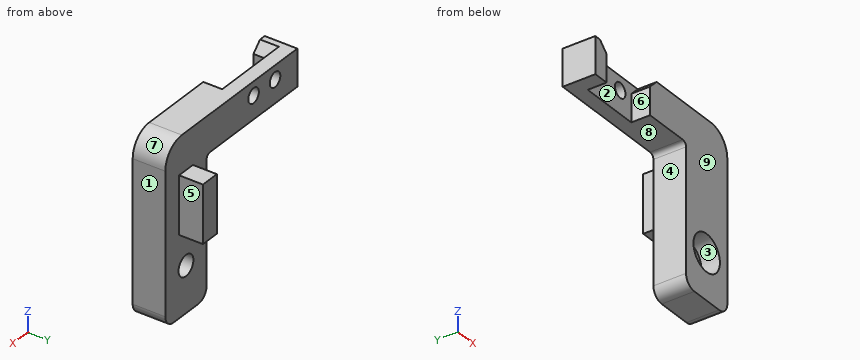
from build123d import *

# Parameters (mm, degrees)
BOSS_EXTRUDE1_DEPTH            = 7.1
SKETCH2_W                      = 4.2
SKETCH2_H                      = 12.5
BOSS_EXTRUDE2_DEPTH            = 5.2
CBORE_FOR_M4_SHCS1_D           = 4.5
CBORE_FOR_M4_SHCS1_CBORE_D     = 8
CBORE_FOR_M4_SHCS1_CBORE_DEPTH = 4
F_3_2_3_2_DIAMETER_HOLE1_D     = 3.2
SKETCH7_W                      = 13.2
SKETCH7_H                      = 8
CUT_EXTRUDE1_DEPTH             = 4.1
FILLET1_R                      = 5
FILLET2_R                      = 2.5
FILLET3_R                      = 1
CHAMFER1_SIZE                  = 2


with BuildPart() as part:
    # Sketch1 → Boss-Extrude1 (new body)
    with BuildSketch(Plane(origin=(0, 0, 0), x_dir=(1, 0, 0), z_dir=(0, 1, 0))):
        Polygon((0, 0), (-12.5, 0), (-12.5, -30), (-40, -30), (-40, -38), (-12.5, -38), (0, -38), align=None)
    extrude(amount=BOSS_EXTRUDE1_DEPTH)

    # Sketch2 → Boss-Extrude2 (add)
    with BuildSketch(Plane(origin=(0, 7.1, 0), x_dir=(1, 0, 0), z_dir=(0, 1, 0))):
        with Locations((-6.25, -23.75)):
            Rectangle(SKETCH2_W, SKETCH2_H)
    extrude(amount=BOSS_EXTRUDE2_DEPTH)

    # CBORE for M4 SHCS1 (through all)
    with Locations(Plane.XZ):
        with Locations((-6.25, 10)):
            CounterBoreHole(CBORE_FOR_M4_SHCS1_D / 2, CBORE_FOR_M4_SHCS1_CBORE_D / 2, CBORE_FOR_M4_SHCS1_CBORE_DEPTH)

    # Ø3.2 (3.2) Diameter Hole1 (through all)
    with Locations(Plane.XZ):
        with Locations((-33.25, 35), (-26.75, 35)):
            Hole(F_3_2_3_2_DIAMETER_HOLE1_D / 2)

    # Sketch7 → Cut-Extrude1 (cut)
    with BuildSketch(Plane.XZ):
        with Locations((-30, 34)):
            Rectangle(SKETCH7_W, SKETCH7_H)
    extrude(amount=-CUT_EXTRUDE1_DEPTH, mode=Mode.SUBTRACT)

    # Fillet1
    fillet1_edges = [part.edges().sort_by_distance(p)[0] for p in [
        (0, 3.55, 38),
    ]]
    fillet(fillet1_edges, radius=FILLET1_R)

    # Fillet2
    fillet2_edges = [part.edges().sort_by_distance(p)[0] for p in [
        (-12.5, 3.55, 0),
        (0, 3.55, 0),
    ]]
    fillet(fillet2_edges, radius=FILLET2_R)

    # Fillet3
    fillet3_edges = [part.edges().sort_by_distance(p)[0] for p in [
        (-12.5, 3.55, 30),
    ]]
    fillet(fillet3_edges, radius=FILLET3_R)

    # Chamfer1
    chamfer1_edges = [part.edges().sort_by_distance(p)[0] for p in [
        (-23.4, 2.05, 38),
        (-36.6, 2.05, 38),
    ]]
    chamfer(chamfer1_edges, length=CHAMFER1_SIZE)


solid = part.part
Geometry: final body of the model. Coordinates: model frame, mm. Face numbers are marked on the shaded views. A direction names the side the tool comes from. Coordinates: 2 decimals unless noted, no trailing zeros. Loops run counter-clockwise (first coordinate to the right, second up) from the corner with the lowest first, then second, coordinate; pieces in that order, holes last. Notation, with made-up numbers: (54, 33) - (97, 33) arc R26 cw to (97, 54) - close; hole circle Ø10 at (79.5, -23). An arc over 180 degrees is marked (long way). Put each result on its own line as item: value. Start each with the question number.
Q1. Cut plane B-B, the plane x = -26.75. Return loops of the section in (y, z).
Q2. Cut plane D-D, the plane x = -6.25. Return loops of the section in (y, z), and give its area (3 significant figures).
Q3. Line query: line 1 (Z direction, x = -6.25, y = 1); line 2 (Z direction, x = -6.25, y = 6); line 3 (Z direction, x = -13.5, y = 1.5). Output: solid intervals per line, ascending.
Q4. Set-up query: the marked faces 5, 6, 7, 8 and 9. Return all of +Z, -Z, +X, -X, +Y, -Y with unobstructed straight access to the full face (end or side cutting, diameter ignored); none if empty.
Q5. Cut plane C-C, the plane y = 5. Return loops of the section in (x, z), and give its area (3 significant figures).
Q6. Pin query (flat end, axial travel): pin 1 Ø5 at (x, z) = (-15.5, 32) entering from +Y; pin 2 Ø2.5 at (y, z) = (9.5, 24) entering from +X; pin 3 Ø1 at (y, z) = (11, 24) entering from -X; pin 4 Ø3.5 at (x, z) = (-6.25, 10) entering from +Y. Return the tip coordinate at first contact, or that it passes through.
Q7. Pull-direction query (X, two-part tool) for the marked faces 1, 2, 3 and 4; classes: released by +X, released by -X, zero draft, split by the parting line, or undercut.
Q8. Cut plane A-A, the plane z = 10. Return loops of the section in (x, y).
Filled sheet:
1. outline: (4.1, 30) - (7.1, 30) - (7.1, 33.4) - (4.1, 33.4) - close; (4.1, 36.6) - (7.1, 36.6) - (7.1, 38) - (4.1, 38) - close
2. outline: (0, 0) - (7.1, 0) - (7.1, 7.75) - (4, 7.75) - (4, 6) - (0, 6) - close; (0, 14) - (4, 14) - (4, 12.25) - (7.1, 12.25) - (7.1, 17.5) - (12.3, 17.5) - (12.3, 30) - (7.1, 30) - (7.1, 38) - (0, 38) - close
2. area: 289 mm²
3. line 1: 0 to 6, 14 to 38
3. line 2: 0 to 7.75, 12.25 to 38
3. line 3: 30 to 38
4. face 5: +Z, -Z, +X, +Y
4. face 6: +Z, -Z, -Y
4. face 7: +Z, +X, +Y, -Y
4. face 8: -Z, -X, +Y, -Y
4. face 9: +Z, -Z, +X, -X, -Y
5. outline: (-40, 30) - (-13.5, 30) arc R1 cw to (-12.5, 29) - (-12.5, 2.5) arc R2.5 ccw to (-10, 0) - (-2.5, 0) arc R2.5 ccw to (0, 2.5) - (0, 33) arc R5 ccw to (-5, 38) - (-40, 38) - close; hole circle Ø3.2 at (-33.25, 35); hole circle Ø3.2 at (-26.75, 35); hole circle Ø4.5 at (-6.25, 10)
5. area: 655 mm²
6. pin 1: y = 7.1
6. pin 2: x = -4.15
6. pin 3: x = -8.35
6. pin 4: through
7. face 1: released by +X
7. face 2: undercut
7. face 3: undercut
7. face 4: released by -X
8. outline: (-12.5, 0) - (-10.25, 0) - (-10.25, 4) - (-8.5, 4) - (-8.5, 7.1) - (-12.5, 7.1) - close; (-4, 4) - (-2.25, 4) - (-2.25, 0) - (0, 0) - (0, 7.1) - (-4, 7.1) - close
